```python
from build123d import *

# Parameters (mm, degrees)
F0_R     = 5
F3_DEPTH = 25
F5_R     = 12.5
F6_DEPTH = 25


with BuildPart() as f2:
    # F1 (on Front) → F2 (revolve)
    with BuildSketch(Plane.XZ):
        Polygon((-31.5, 31.5), (-32.75, 0), (-63.5, 0), (-63.5, -7), (-37.5, -27.5), (-30.5, -27.5), (-30.5, -37.5), (-26, -37.5), (-26, -22.5), (-22, -22.5), (-22, 16.5), (-26, 16.5), (-26, 31.5), align=None)
    revolve(axis=Axis((0, 0, 30.379497), (0, 0, 1)))

    # F0 (on Top) → F3 (cut)
    with BuildSketch(Plane.XY):
        with Locations((-37.5, 37.5)):
            Circle(F0_R)
        with Locations((-37.5, -37.5)):
            Circle(F0_R)
        with Locations((37.5, -37.5)):
            Circle(F0_R)
        with Locations((37.5, 37.5)):
            Circle(F0_R)
    extrude(amount=-F3_DEPTH, mode=Mode.SUBTRACT)

    # F5 (on offset) → F6 (cut)
    with BuildSketch(Plane.XY.offset(-7)):
        with Locations((-37.5, 37.5)):
            Circle(F5_R)
        with Locations((37.5, 37.5)):
            Circle(F5_R)
        with Locations((-37.5, -37.5)):
            Circle(F5_R)
        with Locations((37.5, -37.5)):
            Circle(F5_R)
    extrude(amount=-F6_DEPTH, mode=Mode.SUBTRACT)


solid = f2.part
```
Here's how the part is built. I have some questions about the finished solid (model axes, mm). A direction names the side the tool comes from. Give positions to 0.01 mm unless a question says otherwise; leave off trailing zeros. Write each loop counter-clockwise with the first axis right and the second up, starting at its lowest first coordinate (ties: lowest second). Pieces come first, ordered by that corner, then holes. Notation, with made-up numbers: M 21,57.5 L 45,57.5 A6 ccw 45,61.5 Z; hole C -24.75,42 d6. An arc over 180 degrees is marked long. Put each result on its own line as item: value. Start each with the question number.
Item 1: I need wall thicknesses on L1, parallel to X at y = 0, z = -33.75; L2, parallel to Y at x = 37, z = -4; L3, parallel to X at y = -37, z = -19. Which ranges of each line are inside material? Lowest first, please. Write a range as from..to.
Item 2: Thinking about a two-plate mould opening in X: for faces 1 (the conical face through (-35.81, 14.85, -26.5)), 2 (the flat face through (19, -12, -22.5)), 3 (the flat face through (-22.5, -13.7, -37.5)), which applies, +X half, -X half, draft (parallel to the pull), parting line (faces both ways), or undercut?
Item 3: On a 3-axis mill with a long thin cutter (end or side, diameter ignored), from which of +Z, -Z, +X, -X, +Y, -Y can I reach the whole of each face in a straight line? I mean faces 4 (the flat face through (37, 32, -7)), 5 (the flat face through (-19, -12, 16.5)), 6 (the cylindrical face through (-42.495, -37.28, -3.451)). Say none if no direction works.
Item 4: If we section it at D-D, the plane y = 35.5: Count the separate pieces of the cut face and the enclosed holes in it, then the cut area to 3 significant figures.
Item 5: Will these pins go through, and if not, where does the flat tip stop? pin 1 (1 mm diameter, centred on x = -15.5, z = 9, fed in from +Y); pin 2 (1.5 mm diameter, centred on x = -5.5, z = -16.5, fed in from +Y); pin 3 (5 mm diameter, centred on y = 3, z = 12.5, fed in from -X).
Item 6: If we section it at A-A, the plane x = 0: Write out the boundary of the cut face in (y, z).
Item 7: If we section it at C-C, the plane z = -12.5: Write out the boundary of the cut face in (x, y).
Values:
1. L1: -30.5..-26, 26..30.5
1. L2: -51.61..-42.47, -32.53..32.53, 42.47..51.61
1. L3: -25.01..25.01
2. face 1: parting line
2. face 2: undercut
2. face 3: draft
3. face 4: -Z
3. face 5: +Z
3. face 6: +Z, -Z
4. separate pieces: 3
4. enclosed holes: 0
4. area: 1,590 mm²
5. pin 1: y = 28.71
5. pin 2: y = 52.12
5. pin 3: x = -32.3
6. outline: M -63.5,-7 L -37.5,-27.5 L -30.5,-27.5 L -30.5,-37.5 L -26,-37.5 L -26,-22.5 L -22,-22.5 L -22,16.5 L -26,16.5 L -26,31.5 L -31.5,31.5 L -32.75,0 L -63.5,0 Z; M 22,-22.5 L 26,-22.5 L 26,-37.5 L 30.5,-37.5 L 30.5,-27.5 L 37.5,-27.5 L 63.5,-7 L 63.5,0 L 32.75,0 L 31.5,31.5 L 26,31.5 L 26,16.5 L 22,16.5 Z
7. outline: M -47.72,-30.3 A12.5 cw long -30.3,-47.72 A56.52 ccw 30.3,-47.72 A12.5 cw long 47.72,-30.3 A56.52 ccw 47.72,30.3 A12.5 cw long 30.3,47.72 A56.52 ccw -30.3,47.72 A12.5 cw long -47.72,30.3 A56.52 ccw Z; hole C 0,0 d44
